```python
from build123d import *

# Parameters (mm, degrees)
SKETCH1_R           = 3.048
BOSS_EXTRUDE1_DEPTH = 6.35
SKETCH2_W           = 6.35
SKETCH2_H           = 3.81
SKETCH2_H_2         = 4.445
BOSS_EXTRUDE2_DEPTH = 3.81


with BuildPart() as part:
    # Sketch1 → Boss-Extrude1 (new body)
    with BuildSketch(Plane(origin=(0, 0, 0), x_dir=(0, 0, -1), z_dir=(1, 0, 0))):
        with BuildLine():
            ThreePointArc((0, -9.525), (6.735192091, 6.735192091), (-9.525, 0))
            Line((-9.525, 0), (-21.59, 0))
            Line((-21.59, 0), (-21.59, -9.525))
            Line((-21.59, -9.525), (0, -9.525))
        make_face()
        Circle(SKETCH1_R, mode=Mode.SUBTRACT)
    extrude(amount=BOSS_EXTRUDE1_DEPTH)

    # Sketch2 → Boss-Extrude2 (add)
    with BuildSketch(Plane.ZY):
        with Locations((18.415, -1.905)):
            Rectangle(SKETCH2_W, SKETCH2_H)
        with Locations((18.415, -7.3025)):
            Rectangle(SKETCH2_W, SKETCH2_H_2)
    extrude(amount=BOSS_EXTRUDE2_DEPTH)


solid = part.part
```
Verification items for the finished model (mm, model axes). A direction names the side the tool comes from. Give positions to 0.01 mm unless a question says otherwise; leave off trailing zeros. Order: outer loops, then holes, each group sorted by start corner. A loop starts at its lowest first (then second) coordinate and runs counter-clockwise, first axis right, second up. Notation, with made-up numbers: (31.25, 23) -> (50.25, 23) arc R25 cw to (50.25, 52) -> close; hole circle Ø10 at (77.25, 8). An arc over 180 degrees is marked (long way). One line per item, written item: value.
(1) Sectioned sample at D-D on x = 1. Record the cut outline in (y, z) (3 decimals).
Final values:
outline: (-9.525, 0) arc R9.525 ccw (long way) to (0, 9.525) -> (0, 21.59) -> (-9.525, 21.59) -> close; hole circle Ø6.096 at (0, 0)
(2) Tool access check on faces 4 (the face through (3.13, 3.02, 0.4)), 5 (the face through (-2, -3.81, 18)), 6 (the face through (-2, -2, 15.24)). Record the directions out of +Z, -Z, +X, -X, +Y, -Y that give a thin tool (end or side, any length) a straight path to the whole face; none if there is none.
Final values:
face 4: +X, -X
face 5: +Z, -Z, -X
face 6: -Z, -X, +Y, -Y
(3) Sectioned sample at B-B on y = 1. Record the cut outline in (x, z), then the cut area to 3 significant figures.
Final values:
outline: (0, -9.47) -> (6.35, -9.47) -> (6.35, -2.88) -> (0, -2.88) -> close; (0, 2.88) -> (6.35, 2.88) -> (6.35, 9.47) -> (0, 9.47) -> close
area: 83.7 mm^2
(4) Sectioned sample at C-C on z = 18. Record the cut outline in (x, y) (3 decimals), then the cut area to 3 significant figures.
Final values:
outline: (-3.81, -9.525) -> (6.35, -9.525) -> (6.35, 0) -> (-3.81, 0) -> (-3.81, -3.81) -> (0, -3.81) -> (0, -5.08) -> (-3.81, -5.08) -> close
area: 91.9 mm^2
(5) Scan lines: line 1 along Y through (x, z) = (4, 0) (3 decimals); line 2 along Y through (x, z) = (-2, 17) (3 decimals); line 3 along X through (y, z) = (-7.25, 6). Record each from-to range of solid material in increasing order. Write a range as [from, to].
Final values:
line 1: [-9.525, -3.048], [3.048, 9.525]
line 2: [-9.525, -5.08], [-3.81, 0]
line 3: [0, 6.35]
(6) Draft check along Y on faces 1 (the face through (-2, -5.08, 18)), 2 (the face through (-2, -7, 15.24)), 3 (the face through (2, 0, 15)). Enter one of: pulls with the +Y half, pulls with the -Y half, needs draft (parallel to the pull), parting line crosses it, or undercut.
Final values:
face 1: undercut
face 2: needs draft
face 3: pulls with the +Y half
(7) Sectioned sample at A-A on x = -2. Record the cut outline in (y, z) (3 decimals), then the cut area to 3 significant figures.
Final values:
outline: (-9.525, 15.24) -> (-5.08, 15.24) -> (-5.08, 21.59) -> (-9.525, 21.59) -> close; (-3.81, 15.24) -> (0, 15.24) -> (0, 21.59) -> (-3.81, 21.59) -> close
area: 52.4 mm^2
(8) Gauge pin test, flat ends, axial feed: pin 1 (1.1 mm diameter, centred on x = -2, y = -7.5, fed in from -Z); pin 2 (3 mm diameter, centred on x = -2, z = 18, fed in from +Y). Record the tip position at first contact, or that the pin passes through.
Final values:
pin 1: z = 15.24
pin 2: y = 0
